```python
from build123d import *

# Parameters (mm, degrees)
STRUCTURAL_MEMBER1_DEPTH = 1255
CUT_EXTRUDE1_DEPTH       = 50


with BuildPart() as part:
    # Sketch12 → Structural Member1 (new body)
    with BuildSketch(Plane(origin=(0, 0, 0), x_dir=(-1, 0, 0), z_dir=(0, 0, -1))):
        with BuildLine():
            Line((-18.5, -20), (18.5, -20))
            ThreePointArc((18.5, -20), (19.560660172, -19.560660172), (20, -18.5))
            Line((20, -18.5), (20, 18.5))
            ThreePointArc((20, 18.5), (19.560660172, 19.560660172), (18.5, 20))
            Line((18.5, 20), (-18.5, 20))
            ThreePointArc((-18.5, 20), (-19.560660172, 19.560660172), (-20, 18.5))
            Line((-20, 18.5), (-20, -18.5))
            ThreePointArc((-20, -18.5), (-19.560660172, -19.560660172), (-18.5, -20))
        make_face()
        with BuildLine():
            Line((-18.5, -18.8), (18.5, -18.8))
            ThreePointArc((18.5, -18.8), (18.712132034, -18.712132034), (18.8, -18.5))
            Line((18.8, -18.5), (18.8, 18.5))
            ThreePointArc((18.8, 18.5), (18.712132034, 18.712132034), (18.5, 18.8))
            Line((18.5, 18.8), (-18.5, 18.8))
            ThreePointArc((-18.5, 18.8), (-18.712132034, 18.712132034), (-18.8, 18.5))
            Line((-18.8, 18.5), (-18.8, -18.5))
            ThreePointArc((-18.8, -18.5), (-18.712132034, -18.712132034), (-18.5, -18.8))
        make_face(mode=Mode.SUBTRACT)
    extrude(amount=STRUCTURAL_MEMBER1_DEPTH)

    # Sketch13 → Cut-Extrude1 (cut)
    with BuildSketch(Plane(origin=(0, 20, 0), x_dir=(1, 0, 0), z_dir=(0, 1, 0))):
        Polygon((-20, 1255), (31.574006929, 1203.425993071), (31.574006929, 1272.147428422), align=None)
        Polygon((31.574006929, -17.147428422), (-20, 0), (31.574006929, 51.574006929), align=None)
    extrude(amount=-CUT_EXTRUDE1_DEPTH, mode=Mode.SUBTRACT)


solid = part.part
```
Part model, mm, in its own coordinate system. A direction names the side the tool comes from. Round coordinates to 2 decimals unless told otherwise and drop trailing zeros. Write each loop counter-clockwise with the first axis right and the second up, starting at its lowest first coordinate (ties: lowest second). Pieces come first, ordered by that corner, then holes. Notation, with made-up numbers: M 60,-13.5 L 94,-13.5 A20 cw 94,1.5 Z; hole C 38.25,22 d8. An arc over 180 degrees is marked long. Answer as CSV lines item,"result". Start each with the question number.
1) Which spindle directions (+Z, -Z, +X, -X, +Y, -Y) get a long thin tool onto all of the face, cutting with end or side? Do faces 1 (the face through (20, 0, -619)), 2 (the face through (-18.8, 0, -619)). Say none if no direction does.
2) Band-saw the part on A-A (x = 12). List the corners of the cut face in (y, z), then the cut area to 3 significant figures.
3) Mould opens along Y. For faces 3 (the face through (0, -18.8, -619)), 4 (the face through (-2, -19, -1237)), 5 (the face through (0, 20, -619)) say: +Y half, -Y half, draft (parallel to the pull), parting line (faces both ways), or undercut.
4) Band-saw the part on B-B (y = 2.5). List the corners of the cut face in (x, z).
5) Band-saw the part on C-C (z = -351). List the corners of the cut face in (x, y).
6) Drill centre line: L1, parallel to Y at x = -10.5, z = -831. Where is it in solid material? Low to high.
Worked out:
1,face 1,"+Z, -Z, +X, +Y, -Y"
1,face 2,"+Z, -Z"
2,outline,"M -20,-1223 L -18.8,-1223 L -18.8,-32 L -20,-32 Z; M 18.8,-1223 L 20,-1223 L 20,-32 L 18.8,-32 Z"
2,area,"2,860 mm²"
3,face 3,"undercut"
3,face 4,"draft"
3,face 5,"+Y half"
4,outline,"M -20,-1255 L -18.8,-1253.8 L -18.8,-1.2 L -20,0 Z; M 18.8,-1216.2 L 20,-1215 L 20,-40 L 18.8,-38.8 Z"
5,outline,"M -20,-18.5 A1.5 ccw -18.5,-20 L 18.5,-20 A1.5 ccw 20,-18.5 L 20,18.5 A1.5 ccw 18.5,20 L -18.5,20 A1.5 ccw -20,18.5 Z; hole M -18.8,-18.5 A0.3 ccw -18.5,-18.8 L 18.5,-18.8 A0.3 ccw 18.8,-18.5 L 18.8,18.5 A0.3 ccw 18.5,18.8 L -18.5,18.8 A0.3 ccw -18.8,18.5 Z"
6,L1,"-20 to -18.8, 18.8 to 20"
